The model under review builds one solid part; all positions refer to its coordinate system, in mm. A direction names the side the tool comes from. Round coordinates to 2 decimals unless told otherwise and drop trailing zeros. Order: outer loops, then holes, each group sorted by start corner. A loop starts at its lowest first (then second) coordinate and runs counter-clockwise, first axis right, second up. Notation, with made-up numbers: M -28.75,-11.5 L -1.75,-11.5 A20 cw -1.75,15.5 Z; hole C 27,9 d1. An arc over 180 degrees is marked long. Answer as a JSON object with one key per item and string values. Group by question number.
1) Consider section C-C, the plane y = 9. Write out the cut boundary in (x, z).
2) For faces 1 (the flat face through (20, 0, 2)), 2 (the flat face through (30, 0, 1)), 3 (the flat face through (22, -9, 2)), list the 3-axis set-ups (+Z, -Z, +X, -X, +Y, -Y) from which the entire face can be reached by the end or side of a thin tool; tool diameter is ignored.
3) To check wall thickness, follow line 1 (Y direction, x = 26, z = 0.75); line 2 (X direction, y = -9, z = 2.2); line 3 (Y direction, x = 26, z = 1.7). State the ranges of each line that lie inside material, in increasing order.
4) Insertion check: pin 1 Ø1.5 at (x, z) = (10.5, 1) entering from -Y; pin 2 Ø1.6 at (x, z) = (21.5, 1) entering from +Y; pin 3 Ø3.5 at (x, y) = (26, -1) entering from +Z; pin 4 Ø2 at (y, z) = (0.5, 2) entering from -X. Each pin has a flat end and moves straight along its axis. Give the tip position at first contact, or say it passes through.
5) Consider section D-D, the plane z = 0.65. Write out the cut boundary in (x, y), then the cut area to 3 significant figures.
6) Consider section A-A, the plane z = 2.2. Write out the cut boundary in (x, y), then the cut area to 3 significant figures.
7) The part is to be moulded in two halves that separate along Y. For faces 4 (the flat face through (25, 0, 1.5)), 5 (the flat face through (0, 0, 2)), 6 (the flat face through (26, -12.5, 2)), say which applies: +Y half, -Y half, draft (parallel to the pull), parting line (faces both ways), or undercut.
8) Consider section B-B, the plane x = 26. Write out the cut boundary in (y, z), then the cut area to 3 significant figures.
```python
from build123d import *

# Parameters (mm, degrees)
DODANIE_WYCI_GNI_CIE1_DEPTH = 3.4
DODANIE_WYCI_GNI_CIE2_DEPTH = 1.5
ZAOKR_GLENIE1_R             = 2
SZKIC4_W                    = 8
SZKIC4_H                    = 5
DODANIE_WYCI_GNI_CIE3_DEPTH = 3.4
ZAOKR_GLENIE2_R             = 2
SZKIC6_R                    = 1.15
WYTNIJ_WYCI_GNI_CIE1_DEPTH  = 3.5


with BuildPart() as part:
    # Szkic1 → Dodanie-wyciągnięcie1 (new body)
    with BuildSketch(Plane.XY):
        Polygon((0, 0), (0, 6), (20, 6), (20, -6), (0, -6), align=None)
    extrude(amount=DODANIE_WYCI_GNI_CIE1_DEPTH)

    # Szkic3 → Dodanie-wyciągnięcie2 (add)
    with BuildSketch(Plane.XY):
        Polygon((20, 6), (20, 7.5), (30, 7.5), (30, -7.5), (20, -7.5), (20, -6), align=None)
    extrude(amount=DODANIE_WYCI_GNI_CIE2_DEPTH)

    # Zaokrąglenie1
    # the kernel refuses this fillet: 2 mm, written as the material it adds along each edge
    with BuildSketch(Plane(origin=(20, -6, 0), x_dir=(-1, 0, 0), z_dir=(0, 0, 1))) as zaokr_glenie1_piece_1:
        with BuildLine():
            CenterArc((1.936491673, 2), ZAOKR_GLENIE1_R, 194.477512186, 75.522487814)
            Line((0, 1.5), (0, 0))
            Line((0, 0), (1.936491673, 0))
        make_face()
    extrude(amount=1.5)
    with BuildSketch(Plane(origin=(20, 6, 0), x_dir=(-1, 0, 0), z_dir=(0, 0, 1))) as zaokr_glenie1_piece_2:
        with BuildLine():
            CenterArc((1.936491673, -2), ZAOKR_GLENIE1_R, 90, 75.522487814)
            Line((0, -1.5), (0, 0))
            Line((0, 0), (1.936491673, 0))
        make_face()
    extrude(amount=1.5)
    # the kernel refuses this fillet: 2 mm, written as the material it takes off along each edge
    with BuildSketch(Plane(origin=(0, -6, -5), x_dir=(0, 1, 0), z_dir=(0, 0, 1))) as zaokr_glenie1_2_piece_1:
        with BuildLine():
            CenterArc((ZAOKR_GLENIE1_R, -ZAOKR_GLENIE1_R), ZAOKR_GLENIE1_R, 90, 90)
            Line((0, -ZAOKR_GLENIE1_R), (0, 0))
            Line((0, 0), (ZAOKR_GLENIE1_R, 0))
        make_face()
    extrude(amount=13.4, mode=Mode.SUBTRACT)
    with BuildSketch(Plane(origin=(0, 6, -5), x_dir=(0, -1, 0), z_dir=(0, 0, 1))) as zaokr_glenie1_2_piece_2:
        with BuildLine():
            CenterArc((ZAOKR_GLENIE1_R, ZAOKR_GLENIE1_R), ZAOKR_GLENIE1_R, 180, 90)
            Line((0, ZAOKR_GLENIE1_R), (0, 0))
            Line((0, 0), (ZAOKR_GLENIE1_R, 0))
        make_face()
    extrude(amount=13.4, mode=Mode.SUBTRACT)

    # Szkic4 → Dodanie-wyciągnięcie3 (add)
    with BuildSketch(Plane.XY):
        with Locations((26, 10)):
            Rectangle(SZKIC4_W, SZKIC4_H)
        with Locations((26, -10)):
            Rectangle(SZKIC4_W, SZKIC4_H)
    extrude(amount=DODANIE_WYCI_GNI_CIE3_DEPTH)

    # Zaokrąglenie2
    zaokr_glenie2_edges = [part.edges().sort_by_distance(p)[0] for p in [
        (30, 12.5, 1.7),
        (22, 12.5, 1.7),
        (22, -12.5, 1.7),
        (30, -12.5, 1.7),
    ]]
    fillet(zaokr_glenie2_edges, radius=ZAOKR_GLENIE2_R)

    # Szkic6 → Wytnij-wyciągnięcie1 (cut)
    with BuildSketch(Plane.XY):
        with Locations(Location((26, 9, 0), (0, 0, 180))):
            Circle(SZKIC6_R)
        with Locations((26, -9)):
            Circle(SZKIC6_R)
    extrude(amount=WYTNIJ_WYCI_GNI_CIE1_DEPTH, mode=Mode.SUBTRACT)


solid = part.part
```
Results list:
{
 "1": {"outline": "M 22,0 L 24.85,0 L 24.85,3.4 L 22,3.4 Z; M 27.15,0 L 30,0 L 30,3.4 L 27.15,3.4 Z"},
 "2": {"face 1": "+Z, +X, +Y, -Y", "face 2": "+Z, -Z, +X, +Y, -Y", "face 3": "+Z, -Z, -X, -Y"},
 "3": {"line 1": "-12.5 to -10.15, -7.85 to 7.85, 10.15 to 12.5", "line 2": "22 to 24.85, 27.15 to 30", "line 3": "-12.5 to -10.15, -7.85 to -7.5, 7.5 to 7.85, 10.15 to 12.5"},
 "4": {"pin 1": "y = -6", "pin 2": "y = 11.55", "pin 3": "z = 1.5", "pin 4": "x = 0"},
 "5": {"outline": "M 0,-4 A2 ccw 2,-6 L 18.06,-6 A2 cw 20,-7.5 L 22,-7.5 L 22,-10.5 A2 ccw 24,-12.5 L 28,-12.5 A2 ccw 30,-10.5 L 30,10.5 A2 ccw 28,12.5 L 24,12.5 A2 ccw 22,10.5 L 22,7.5 L 20,7.5 A2 cw 18.06,6 L 2,6 A2 ccw 0,4 Z; hole C 26,-9 d2.3; hole C 26,9 d2.3", "area": "458 mm^2"},
 "6": {"outline": "M 0,-4 A2 ccw 2,-6 L 20,-6 L 20,6 L 2,6 A2 ccw 0,4 Z; M 22,-10.5 A2 ccw 24,-12.5 L 28,-12.5 A2 ccw 30,-10.5 L 30,-7.5 L 22,-7.5 Z; M 22,7.5 L 30,7.5 L 30,10.5 A2 ccw 28,12.5 L 24,12.5 A2 ccw 22,10.5 Z; hole C 26,-9 d2.3; hole C 26,9 d2.3", "area": "307 mm^2"},
 "7": {"face 4": "undercut", "face 5": "draft", "face 6": "-Y half"},
 "8": {"outline": "M -12.5,0 L -10.15,0 L -10.15,3.4 L -12.5,3.4 Z; M -7.85,0 L 7.85,0 L 7.85,3.4 L 7.5,3.4 L 7.5,1.5 L -7.5,1.5 L -7.5,3.4 L -7.85,3.4 Z; M 10.15,0 L 12.5,0 L 12.5,3.4 L 10.15,3.4 Z", "area": "40.9 mm^2"}
}
